The listing builds one solid part. Answer for the finished solid, in the listing's coordinates (mm). A direction names the side the tool comes from. Give positions to 0.01 mm unless a question says otherwise; leave off trailing zeros. Loops run counter-clockwise (first coordinate to the right, second up) from the corner with the lowest first, then second, coordinate; pieces in that order, holes last. Notation, with made-up numbers: (71, 73) - (120, 73) arc R30 ccw to (120, 95) - close; hole circle Ø7 at (-23.75, -35.5). An arc over 180 degrees is marked (long way). Write each question's results on one line, items separated by ' | '.
from build123d import *

# Parameters (mm, degrees)
EXTRUDE_1_DEPTH       = 4
SKETCH_4_R            = 1
EXTRUDE_2_DEPTH       = 3
CHAMFER_1_SIZE        = 0.25
HOLE_WIZARD_M23_D     = 1.6
HOLE_WIZARD_M23_DEPTH = 4
HOLE_WIZARD_M23_TIP   = 0.480688495


with BuildPart() as part:
    # Эскиз1 → Бобышка-Вытянуть1 (new body)
    with BuildSketch(Plane(origin=(0, 0, 0), x_dir=(1, 0, 0), z_dir=(0, 1, 0))):
        Polygon((0, 1.5), (-1.299038106, 0.75), (-1.299038106, -0.75), (0, -1.5), (1.299038106, -0.75), (1.299038106, 0.75), align=None)
    extrude(amount=EXTRUDE_1_DEPTH)

    # Эскиз4 → Бобышка-Вытянуть2 (add)
    with BuildSketch(Plane.XZ):
        with Locations(Location((0, 0, 0), (0, 0, 270))):
            Circle(SKETCH_4_R)
    extrude(amount=EXTRUDE_2_DEPTH)

    # Фаска1
    chamfer_1_edges = [part.edges().sort_by_distance(p)[0] for p in [
        (0, -3, 1),
    ]]
    chamfer(chamfer_1_edges, length=CHAMFER_1_SIZE)

    # Отверстие обработанное метчиком M23
    with Locations(Plane(origin=(0, 4, 0), x_dir=(1, 0, 0), z_dir=(0, 1, 0))):
        with Locations((0, 0)):
            Hole(HOLE_WIZARD_M23_D / 2, depth=HOLE_WIZARD_M23_DEPTH)
            with Locations((0, 0, -(HOLE_WIZARD_M23_DEPTH + HOLE_WIZARD_M23_TIP / 2))):  # 118° drill point
                Cone(0, HOLE_WIZARD_M23_D / 2, HOLE_WIZARD_M23_TIP, mode=Mode.SUBTRACT)


solid = part.part
Item 1: For faces 5 (the face through (0.66, 1.97, -1.12)), 6 (the face through (-1, -1, 0)), determine the directions among +Z, -Z, +X, -X, +Y, -Y from which every point of the face is accessible in a straight line to the end or side of a thin tool.
Values found:
face 5: -Z, +X, +Y, -Y | face 6: -Y
Item 2: Flat-ended cylindrical pins translate along their axes: P1, Ø1.5, axis at x = -1, z = 0, coming from the -Y side; P2, Ø1, axis at x = -1, y = 0, coming from the +Z side; P3, Ø1.4, axis at x = 0, z = 0, coming from the +Y side. Find the tip coordinate at first contact, or state that the pin passes through.
Values found:
P1: stops at y = -3 | P2: stops at z = 1.21 | P3: stops at y = -0.06
Item 3: For a pull along X with two mould halves and no side action, classify faces 1 (the face through (0.63, 1.97, 0.49)), 2 (the face through (1.299, 2, 0)), 3 (the face through (-0.1, -0.4, -0.09)), 4 (the face through (-0.64, 1.97, -1.13)) as released by +X, released by -X, zero draft, split by the parting line, or undercut.
Values found:
face 1: undercut | face 2: released by +X | face 3: undercut | face 4: released by -X
Item 4: A cutting plane is placed at A-A, the plane y = 2. Determine the outline of the cut face in (x, z), plus the area to 3 significant figures.
Values found:
outline: (-1.3, -0.75) - (0, -1.5) - (1.3, -0.75) - (1.3, 0.75) - (0, 1.5) - (-1.3, 0.75) - close; hole circle Ø1.6 at (0, 0) | area: 3.84 mm²
Item 5: Find the intervals of material crossed by line 1 along Y through (x, z) = (-0.35, 1.15); line 2 along X through (y, z) = (1.25, 0.4); line 3 along Z through (x, y) = (0.25, 0.5), in increasing order. Write a range as [from, to].
Values found:
line 1: y = [0, 4] | line 2: x = [-1.3, -0.69], [0.69, 1.3] | line 3: z = [-1.36, -0.76], [0.76, 1.36]
